The drawing under review shows one solid part. Ordinate dimensions are in mm from its lowest x, y, z. A direction names the side the tool comes from. Round coordinates to 2 decimals unless told otherwise and drop trailing zeros. Loops run counter-clockwise (first coordinate to the right, second up) from the corner with the lowest first, then second, coordinate; pieces in that order, holes last. Notation, with made-up numbers: (-37, 12) - (22, 12) arc R18 cw to (22, 33) - close; hole circle Ø9 at (-21, 25). An arc over 180 degrees is marked (long way). Answer as CSV lines item,"result".
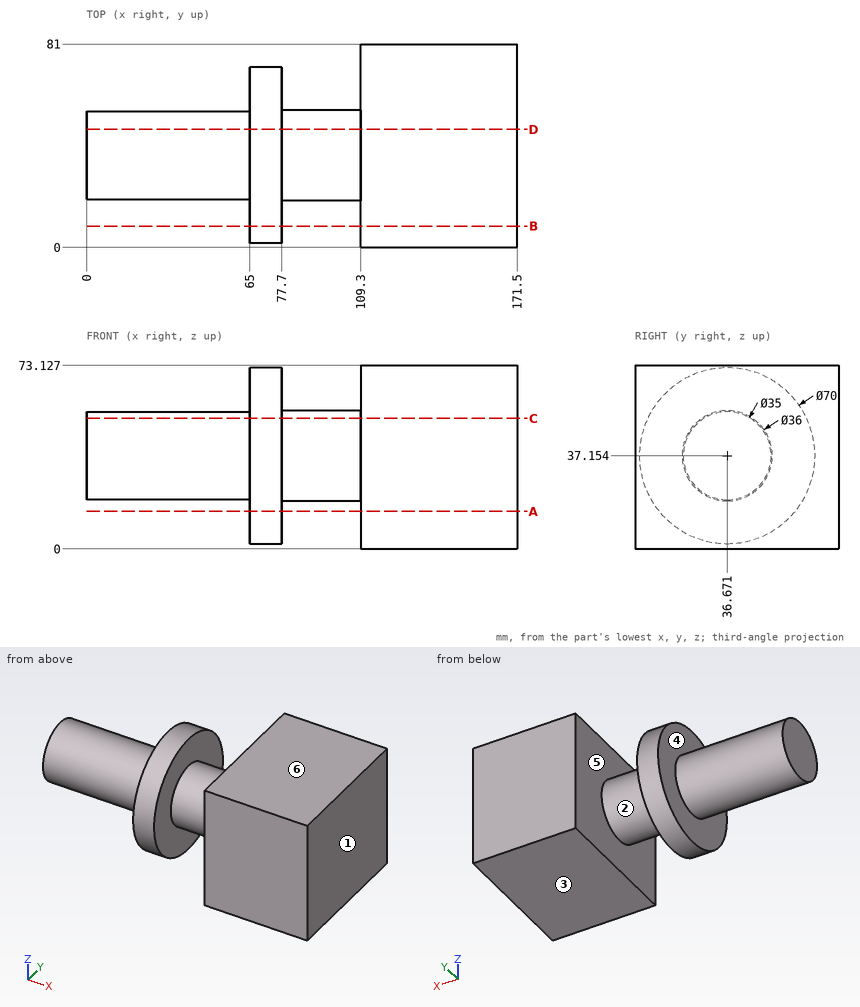
1. Wall thickness on probe 1 along X at (y, z) = (54, 10.5); probe 2 along X at (y, z) = (65, 8); probe 3 along Z at (x, y) = (38.5, 31): over which ranges is each line inside the solid? List them lowest first.
Numbers:
probe 1,"x = 65 to 77.7, 109.3 to 171.5"
probe 2,"x = 109.3 to 171.5"
probe 3,"z = 20.6 to 53.71"
2. Tool access review of the marked faces 4, 5 and 6: name each direction out of +Z, -Z, +X, -X, +Y, -Y from which nothing blocks a thin tool from reaching the whole face with its end or side.
Numbers:
face 4,"-X"
face 5,"none"
face 6,"+Z, +X, -X, +Y, -Y"
3. Draft analysis for pull direction X (two halves, no side actions). For the marked faces 1, 2 and 3, state which applies: +X half, -X half, draft (parallel to the pull), parting line (faces both ways), or undercut.
Numbers:
face 1,"+X half"
face 2,"undercut"
face 3,"draft"
4. Take a section at B-B (y = 8.5). State the section outline as (x, z) points.
Numbers:
outline,"(65, 16.38) - (77.7, 16.38) - (77.7, 57.92) - (65, 57.92) - close; (109.3, 0) - (171.5, 0) - (171.5, 73.13) - (109.3, 73.13) - close"
5. Take a section at D-D (y = 47). State the section outline as (x, z) points (1 decimal).
Numbers:
outline,"(0, 23) - (65, 23) - (65, 3.7) - (77.7, 3.7) - (77.7, 22.4) - (109.3, 22.4) - (109.3, 0) - (171.5, 0) - (171.5, 73.1) - (109.3, 73.1) - (109.3, 51.9) - (77.7, 51.9) - (77.7, 70.6) - (65, 70.6) - (65, 51.3) - (0, 51.3) - close"
6. Take a section at A-A (z = 15). State the section outline as (x, y) points (3 decimals).
Numbers:
outline,"(65, 9.575) - (77.7, 9.575) - (77.7, 63.767) - (65, 63.767) - close; (109.3, 0) - (171.5, 0) - (171.5, 81) - (109.3, 81) - close"
7. Take a section at C-C (z = 52). State the section outline as (x, y) points.
Numbers:
outline,"(0, 27.41) - (65, 27.41) - (65, 4.98) - (77.7, 4.98) - (77.7, 26.49) - (109.3, 26.49) - (109.3, 0) - (171.5, 0) - (171.5, 81) - (109.3, 81) - (109.3, 46.85) - (77.7, 46.85) - (77.7, 68.37) - (65, 68.37) - (65, 45.94) - (0, 45.94) - close"
8. Clearance check with flat-ended pins moving along their axes: pin 1 (4 mm diameter, centred on x = 47, z = 34.5, fed in from -Y); pin 2 (1.5 mm diameter, centred on x = 105.5, z = 20, fed in from -Y); pin 3 (6 mm diameter, centred on x = 61, y = 43, fed in from -Z); pin 4 (8 mm diameter, centred on y = 54, z = 25.5, fed in from -X). State where each tip first meets the part, or that it passes through.
Numbers:
pin 1,"stops at y = 19.18"
pin 2,"stops at y = 29.26"
pin 3,"stops at z = 19.97"
pin 4,"stops at x = 0"
